Check sheet for the modelled part. Datum: model origin and axes. Units: mm. Face numbers are marked on the shaded views. Round coordinates to 2 decimals unless told otherwise and drop trailing zeros. Loops run counter-clockwise (first coordinate to the right, second up) from the corner with the lowest first, then second, coordinate; pieces in that order, holes last. Notation, with made-up numbers: (22, 4) - (36, 4) arc R31 cw to (36, 35) - close; hole circle Ø9 at (15.25, 36). An arc over 180 degrees is marked (long way). Answer in a Markdown table with one row per item. Add a question column.
(1) Cross-section at A-A on z = 202.5. Enter the section's corners in (x, y), then the cut area to 4 significant figures.
(2) Thickness scan on line 1 along X through (y, z) = (21, -95); line 2 along Y through (x, z) = (519.5, -44); line 3 along Z through (x, y) = (-341, -138.5). Record the ranges inside material, lowest first.
(3) Gauge pin test, flat ends, axial feed: pin 1 (22.5 mm diameter, centred on x = -533.5, z = 167, fed in from -Y); pin 2 (2.5 mm diameter, centred on y = 2.5, z = 148, fed in from -X); pin 3 (5.5 mm diameter, centred on y = -286, z = 526.5, fed in from +X). Record the tip position at first contact, or that the pin passes through.
(4) Cross-section at C-C on x = -101. Enter the section's corners in (y, z).
(5) Mould release check, pull along Y, two halves, no side actions. Record for the marked faces 1 and 2: +Y half, -Y half, draft (parallel to the pull), parting line (faces both ways), or undercut.
(6) Cross-section at B-B on x = -520.5. Enter the section's corners in (y, z), then the cut area to 3 significant figures.
(7) Cross-section at D-D on y = -330. Enter the section's corners in (x, z).
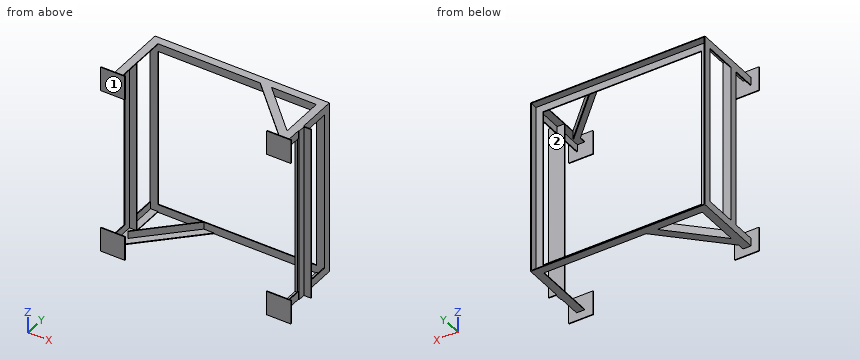
from build123d import *

# Parameters (mm, degrees)
SKETCH_1_W       = 1100
SKETCH_1_H       = 1100
SKETCH_1_W_2     = 1000
SKETCH_1_H_2     = 1000
EXTRUDE_1_DEPTH  = 5
SKETCH_2_W       = 1100
SKETCH_2_H       = 1100
SKETCH_2_W_2     = 1090
SKETCH_2_H_2     = 1090
EXTRUDE_2_DEPTH  = 45
EXTRUDE_3_DEPTH  = 400
SKETCH_4_W       = 152.5
SKETCH_4_H       = 152.5
EXTRUDE_4_DEPTH  = 5
EXTRUDE_6_REACH  = 1355.154
EXTRUDE_7_DEPTH  = 5
EXTRUDE_8_DEPTH  = 45
EXTRUDE_9_DEPTH  = 5
EXTRUDE_10_DEPTH = 45
EXTRUDE_11_DEPTH = 1100


with BuildPart() as part:
    # Эскиз1 → Бобышка-Вытянуть1 (new body)
    with BuildSketch(Plane(origin=(0, 0, 0), x_dir=(1, 0, 0), z_dir=(0, 1, 0))):
        Rectangle(SKETCH_1_W, SKETCH_1_H)
        Rectangle(SKETCH_1_W_2, SKETCH_1_H_2, mode=Mode.SUBTRACT)
    extrude(amount=EXTRUDE_1_DEPTH)

    # Эскиз2 → Бобышка-Вытянуть2 (add)
    with BuildSketch(Plane.XZ.offset(-5)):
        Rectangle(SKETCH_2_W, SKETCH_2_H)
        Rectangle(SKETCH_2_W_2, SKETCH_2_H_2, mode=Mode.SUBTRACT)
    extrude(amount=-EXTRUDE_2_DEPTH)

    # Эскиз3 → Бобышка-Вытянуть3 (add)
    with BuildSketch(Plane.XZ):
        Polygon((550, 550), (500, 550), (500, 545), (545, 545), (545, 500), (550, 500), align=None)
        Polygon((545, -500), (545, -545), (500, -545), (500, -550), (550, -550), (550, -500), align=None)
        Polygon((-550, -550), (-500, -550), (-500, -545), (-545, -545), (-545, -500), (-550, -500), align=None)
        Polygon((-545, 500), (-545, 545), (-500, 545), (-500, 550), (-550, 550), (-550, 500), align=None)
    extrude(amount=EXTRUDE_3_DEPTH)

    # Эскиз4 → Бобышка-Вытянуть4 (add)
    with BuildSketch(Plane.XZ.offset(400)):
        with Locations((523.75, 523.75)):
            Rectangle(SKETCH_4_W, SKETCH_4_H)
        with Locations((523.75, -523.75)):
            Rectangle(SKETCH_4_W, SKETCH_4_H)
        with Locations((-523.75, -523.75)):
            Rectangle(SKETCH_4_W, SKETCH_4_H)
        with Locations((-523.75, 523.75)):
            Rectangle(SKETCH_4_W, SKETCH_4_H)
    extrude(amount=-EXTRUDE_4_DEPTH)

    # Бобышка-Вытянуть6: up to this face of the body (flat: up to its plane)
    extrude_6_end = Plane(part.part.faces().sort_by_distance((522.5, -197.5, 545))[0])
    # Эскиз6 → Бобышка-Вытянуть6 (add, up to the picked face)
    with BuildSketch(Plane.XY.offset(-545), mode=Mode.PRIVATE) as extrude_6_sk1:
        Polygon((500, -200), (550, -200), (550, -250), (545, -250), (545, -205), (500, -205), align=None)
    extrude_6_tool1 = split(extrude(extrude_6_sk1.sketch, amount=EXTRUDE_6_REACH, mode=Mode.PRIVATE), bisect_by=extrude_6_end, keep=Keep.BOTH, mode=Mode.PRIVATE)
    # Эскиз6 → Бобышка-Вытянуть6 (add, up to the picked face)
    with BuildSketch(Plane.XY.offset(-545), mode=Mode.PRIVATE) as extrude_6_sk2:
        Polygon((-545, -250), (-545, -205), (-500, -205), (-500, -200), (-550, -200), (-550, -250), align=None)
    extrude_6_tool2 = split(extrude(extrude_6_sk2.sketch, amount=EXTRUDE_6_REACH, mode=Mode.PRIVATE), bisect_by=extrude_6_end, keep=Keep.BOTH, mode=Mode.PRIVATE)
    add(extrude_6_tool1.solids().sort_by(Axis((525, -200.707107, -545), (0, 0, 1)))[0])
    add(extrude_6_tool2.solids().sort_by(Axis((-545.707107, -227.5, -545), (0, 0, 1)))[0])

    # Эскиз7 → Бобышка-Вытянуть7 (add)
    with BuildSketch(Plane.XY.offset(550)):
        Polygon((146.446609407, 0), (217.157287525, 0), (500, -282.842712475), (500, -353.553390593), align=None)
    extrude(amount=-EXTRUDE_7_DEPTH)

    # Эскиз8 → Бобышка-Вытянуть8 (add)
    with BuildSketch(Plane(origin=(0, 0, 545), x_dir=(-1, 0, 0), z_dir=(0, 0, -1))):
        Polygon((-217.157287525, 0), (-210.086219714, 0), (-500, -289.913780286), (-500, -282.842712475), align=None)
    extrude(amount=EXTRUDE_8_DEPTH)

    # Эскиз9 → Бобышка-Вытянуть9 (add)
    with BuildSketch(Plane(origin=(0, 0, -550), x_dir=(-1, 0, 0), z_dir=(0, 0, -1))):
        Polygon((146.446609407, 0), (500, -353.553390593), (500, -282.842712475), (217.157287525, 0), align=None)
    extrude(amount=-EXTRUDE_9_DEPTH)

    # Эскиз10 → Бобышка-Вытянуть10 (add)
    with BuildSketch(Plane.XY.offset(-545)):
        Polygon((-217.157287525, 0), (-210.086219714, 0), (-500, -289.913780286), (-500, -282.842712475), align=None)
    extrude(amount=EXTRUDE_10_DEPTH)

    # Эскиз11 → Бобышка-Вытянуть11 (add)
    with BuildSketch(Plane.XY.offset(550)):
        Polygon((550, -250), (555, -250), (555, -205), (600, -205), (600, -200), (550, -200), align=None)
    extrude(amount=-EXTRUDE_11_DEPTH)


solid = part.part
Answers:
| question | item | result |
|---|---|---|
| 1 | outline | (-550, -250) - (-545, -250) - (-545, -205) - (-500, -205) - (-500, -200) - (-550, -200) - close; (-550, 0) - (-500, 0) - (-500, 5) - (-545, 5) - (-545, 50) - (-550, 50) - close; (500, -205) - (545, -205) - (545, -250) - (555, -250) - (555, -205) - (600, -205) - (600, -200) - (500, -200) - close; (500, 0) - (550, 0) - (550, 50) - (545, 50) - (545, 5) - (500, 5) - close |
| 1 | area | 2,375 mm^2 |
| 2 | line 1 | x = -550 to -545, 545 to 550 |
| 2 | line 2 | y = -205 to -200, 0 to 5 |
| 2 | line 3 | z = -550 to -545 |
| 3 | pin 1 | stops at y = -205 |
| 3 | pin 2 | stops at x = -550 |
| 3 | pin 3 | stops at x = 550 |
| 4 | outline | (0, -550) - (50, -550) - (50, -545) - (5, -545) - (5, -500) - (0, -500) - close; (0, 500) - (5, 500) - (5, 545) - (50, 545) - (50, 550) - (0, 550) - close |
| 5 | face 1 | -Y half |
| 5 | face 2 | undercut |
| 6 | outline | (-400, -600) - (-395, -600) - (-395, -550) - (50, -550) - (50, -545) - (5, -545) - (5, 545) - (50, 545) - (50, 550) - (-395, 550) - (-395, 600) - (-400, 600) - (-400, 447.5) - (-395, 447.5) - (-395, 545) - (-205, 545) - (-205, -545) - (-395, -545) - (-395, -447.5) - (-400, -447.5) - close; hole (-200, -545) - (0, -545) - (0, 545) - (-200, 545) - close |
| 6 | area | 16,900 mm^2 |
| 7 | outline | (-550, -550) - (-476.45, -550) - (-476.45, -545) - (-545, -545) - (-545, -500) - (-550, -500) - close; (-550, 500) - (-545, 500) - (-545, 545) - (-500, 545) - (-500, 550) - (-550, 550) - close; (476.45, 545) - (545, 545) - (545, 500) - (550, 500) - (550, 550) - (476.45, 550) - close; (500, -550) - (550, -550) - (550, -500) - (545, -500) - (545, -545) - (500, -545) - close |
